from build123d import *

# Parameters (mm, degrees)
F1_DEPTH = 1.58
F2_R     = 2
F3_D     = 3.2


with BuildPart() as f1:
    # F0 (on Top) → F1 (new body)
    with BuildSketch(Plane.XY):
        Polygon((13.5, -40.25), (35, -40.25), (35, 40.25), (-35, 40.25), (-35, -40.25), (-23.5, -40.25), (-21.5, -42.25), (11.5, -42.25), align=None)
    extrude(amount=F1_DEPTH)

    # F2
    f2_edges = [f1.edges().sort_by_distance(p)[0] for p in [
        (-35, 40.25, 0.79),
        (35, 40.25, 0.79),
        (-35, -40.25, 0.79),
        (35, -40.25, 0.79),
    ]]
    fillet(f2_edges, radius=F2_R)

    # F3 (through all)
    with Locations(Plane(origin=(0, 0, 0), x_dir=(1, 0, 0), z_dir=(0, 0, -1))):
        with Locations((-24.13, -12.32), (24.13, -11.05), (8.89, 39.75)):
            Hole(F3_D / 2)


solid = f1.part
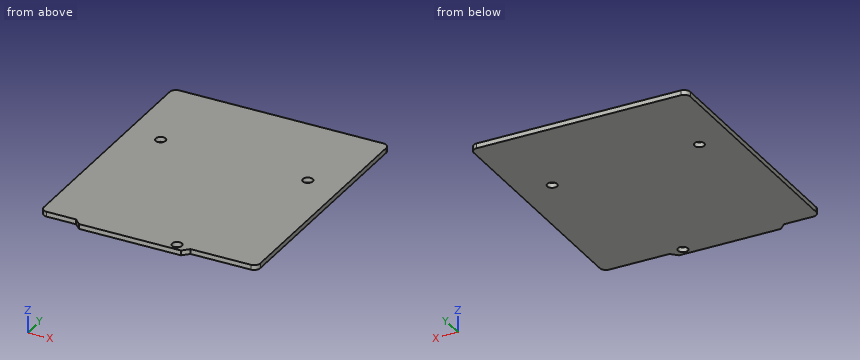
Can you work these out from the model? Positions are in its coordinate system, mm. Round coordinates to 2 decimals unless told otherwise and drop trailing zeros. Write each loop counter-clockwise with the first axis right and the second up, starting at its lowest first coordinate (ties: lowest second). Pieces come first, ordered by that corner, then holes. Notation, with made-up numbers: M -6,38 L 52,38 A38 ccw 52,77 Z; hole C 7,-6.75 d2. An arc over 180 degrees is marked long. Use a Markdown table: item, result.
Item 1: I want a section at B-B (z = 0.95). List the corners of the cut face in (x, y) for me.
Found:
| item | result |
|---|---|
| outline | M -35,-38.25 A2 ccw -33,-40.25 L -23.5,-40.25 L -21.5,-42.25 L 11.5,-42.25 L 13.5,-40.25 L 33,-40.25 A2 ccw 35,-38.25 L 35,38.25 A2 ccw 33,40.25 L -33,40.25 A2 ccw -35,38.25 Z; hole C -24.13,12.32 d3.2; hole C 8.89,-39.75 d3.2; hole C 24.13,11.05 d3.2 |
Item 2: If I drill on line 1 along Y through (x, z) = (24.13, 0.4); line 2 along X through (y, z) = (12.32, 0.7); line 3 along X through (y, z) = (11.05, 1.2), over which ranges is the centre line in solid material (lowest first)? Write a range as [from, to].
Found:
| item | result |
|---|---|
| line 1 | y = [-40.25, 9.45], [12.65, 40.25] |
| line 2 | x = [-35, -25.73], [-22.53, 23.16], [25.1, 35] |
| line 3 | x = [-35, -25.1], [-23.16, 22.53], [25.73, 35] |
Item 3: I want a section at A-A (x = 8.89). List the corners of the cut face in (y, z) for me.
Found:
| item | result |
|---|---|
| outline | M -42.25,0 L -41.35,0 L -41.35,1.58 L -42.25,1.58 Z; M -38.15,0 L 40.25,0 L 40.25,1.58 L -38.15,1.58 Z |
Item 4: I want a section at C-C (x = 24.13). List the corners of the cut face in (y, z) for me.
Found:
| item | result |
|---|---|
| outline | M -40.25,0 L 9.45,0 L 9.45,1.58 L -40.25,1.58 Z; M 12.65,0 L 40.25,0 L 40.25,1.58 L 12.65,1.58 Z |
Item 5: For pin 1 Ø5 at (x, y) = (-24.13, 12.32) entering from +Z; pin 2 Ø0.8 at (x, z) = (22, 1) entering from -Y, each with a flat end and sliding along its axis, tell me the tip position at first contact or that it passes through.
Found:
| item | result |
|---|---|
| pin 1 | stops at z = 1.58 |
| pin 2 | stops at y = -40.25 |
